Could you check a few things on this model? Use its own coordinates, in mm. Face numbers are marked on the shaded views. A direction names the side the tool comes from. Coordinates: 2 decimals unless noted, no trailing zeros. Order: outer loops, then holes, each group sorted by start corner. A loop starts at its lowest first (then second) coordinate and runs counter-clockwise, first axis right, second up. Notation, with made-up numbers: (-11, 26) -> (36, 26) arc R13 ccw to (36, 43) -> close; hole circle Ø11 at (46.5, 6.5). An arc over 180 degrees is marked (long way). Return JSON: item names as keys, results as strings. Group by question number.
Autodesk Inventor part; units mm, degrees
ref_plane "YZ Plane" through (0, 0, 0) normal (1, 0, 0) x (0, 1, 0)
ref_plane "XZ Plane" through (0, 0, 0) normal (0, 1, 0) x (-1, 0, 0)
ref_plane "XY Plane" through (0, 0, 0) normal (0, 0, 1) x (1, 0, 0)
sketch "Sketch1" plane through (0, 0, 0) normal (0, 1, 0) x (-1, 0, 0)
  line L0 (-1.3568, -2.35) -> (-2.7135, 0)
  line L1 (-2.7135, 0) -> (-1.3568, 2.35)
  line L2 (-1.3568, 2.35) -> (1.3568, 2.35)
  line L3 (1.3568, 2.35) -> (2.7135, 0)
  line L4 (2.7135, 0) -> (1.3568, -2.35)
  line L5 (1.3568, -2.35) -> (-1.3568, -2.35)
  point P0 (0, 0)
  point P1 (0, 0)
  dimension "d13" = 4.7
extrude "Extrusion1" add sketch "Sketch1" along normal blind 5
sketch "Sketch3" plane through (0, 0, 0) normal (0, -1, 0) x (1, 0, 0)
  circle A0 centre (0, 0) radius 1.35
  dimension "d12" = 2.7
extrude "Extrusion2" add sketch "Sketch3" along normal blind 5
sketch "Sketch6" plane through (0, 5, 0) normal (0, 1, 0) x (1, 0, 0)
  point P0 (0, 0)
  point P1 (0, 0)
hole "Hole1" at (0, 5, 0) direction (0, -1, 0) diameter 2.5 depth 4 tip angle 118
properties part number "distances"
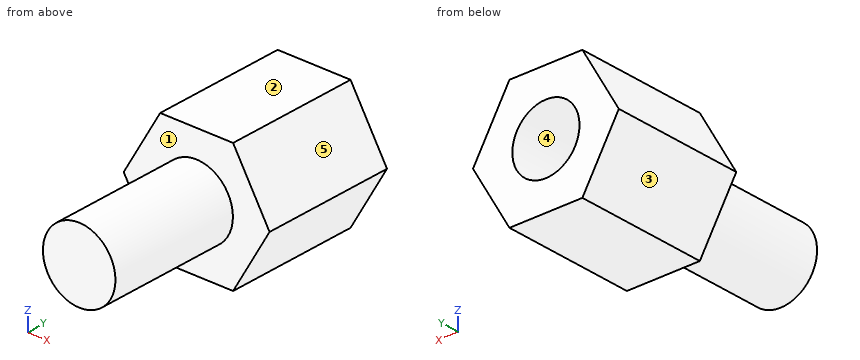
Q1. On a 3-axis mill with a long thin cutter (end or side, diameter ignored), from which of +Z, -Z, +X, -X, +Y, -Y can I reach the whole of each face in a straight line? I mean the marked faces 1 and 2. Say none if no direction works.
Q2. I'm going to push a flat-ended pin straight in: pin 1 Ø1.5 at (x, y) = (-1.5, 1) entering from -Z. Where does the tip first touch, or does it pass through?
Q3. I want a section at A-A on y = 1.5. Please give me the cut outline in (x, z).
Q4. I want a section at B-B on z = -1.9. Please give me the cut outline in (x, y).
Q5. I need wall thicknesses on line 1 along Z through (x, y) = (0, 2.2); line 2 along Y through (x, z) = (-0.85, -1.8); line 3 along X through (y, z) = (3.75, -1.1). Which ranges of each line are inside material? Lowest first, please. Write a range as from..to.
Q6. We'd pull the mould along Z, two halves only. Please class the marked faces 3, 4 and 5: pulls with the +Z half, pulls with the -Z half, needs draft (parallel to the pull), parting line crosses it, or undercut.
Response values:
{
 "1": {"face 1": "-Y", "face 2": "+Z, +X, -X, +Y, -Y"},
 "2": {"pin 1": "stops at z = -2.35"},
 "3": {"outline": "(-2.71, 0) -> (-1.36, -2.35) -> (1.36, -2.35) -> (2.71, 0) -> (1.36, 2.35) -> (-1.36, 2.35) -> close; hole circle Ø2.5 at (0, 0)"},
 "4": {"outline": "(-1.62, 0) -> (1.62, 0) -> (1.62, 5) -> (-1.62, 5) -> close"},
 "5": {"line 1": "z = -2.35..-1.25, 1.25..2.35", "line 2": "y = 0..5", "line 3": "x = -2.08..-0.59, 0.59..2.08"},
 "6": {"face 3": "pulls with the -Z half", "face 4": "undercut", "face 5": "pulls with the +Z half"}
}
